Verification items for the finished model (mm, model axes). A direction names the side the tool comes from. Round coordinates to 2 decimals unless told otherwise and drop trailing zeros. Order: outer loops, then holes, each group sorted by start corner. A loop starts at its lowest first (then second) coordinate and runs counter-clockwise, first axis right, second up. Notation, with made-up numbers: (47, 0) -> (79, 0) arc R32 cw to (79, 28) -> close; hole circle Ø2 at (-12.75, 42). An arc over 180 degrees is marked (long way). Put each result on its own line as item: value.
```python
from build123d import *

# Parameters (mm, degrees)
CUT_EXTRUDE_1_DEPTH = 80.296910406
CUT_EXTRUDE_2_DEPTH = 4


with BuildPart() as part:
    # Sketch 1 → Revolve 1 (revolve)
    with BuildSketch(Plane.XY, mode=Mode.PRIVATE) as revolve_1_sk:
        with BuildLine():
            Line((9, 8), (2.5, 8))
            Line((2.5, 8), (2.5, 0))
            Line((2.5, 0), (56, 0))
            Line((56, 0), (56, 0.4))
            ThreePointArc((56, 0.4), (54.4, 2), (56, 3.6))
            Line((56, 3.6), (56, 4))
            Line((56, 4), (9, 4))
            Line((9, 4), (9, 8))
        make_face()
    revolve(revolve_1_sk.sketch.rotate(Axis((0, 4, 0), (0, 1, 0)), 90), axis=Axis((0, 4, 0), (0, 1, 0)))

    # Sketch 2 → Cut-Extrude 1 (cut, through all)
    with BuildSketch(Plane(origin=(0, 4, 0), x_dir=(1, 0, 0), z_dir=(0, 1, 0))):
        with BuildLine():
            ThreePointArc((24.385885739, -45.927427282), (40.999913751, -31.984481744), (50.480932382, -12.476997468))
            Line((50.480932382, -12.476997468), (8.559508647, 2.781152949))
            Line((8.559508647, 2.781152949), (24.385885739, -45.927427282))
        make_face()
        with BuildLine():
            ThreePointArc((-36.143925877, -37.384711076), (-17.749379666, -48.876983555), (3.733136252, -51.865823947))
            Line((3.733136252, -51.865823947), (5.290067271, -7.281152949))
            Line((5.290067271, -7.281152949), (-36.143925877, -37.384711076))
        make_face()
        with BuildLine():
            Line((-5.290067271, -7.281152949), (-46.724060418, 22.822405177))
            ThreePointArc((-46.724060418, 22.822405177), (-51.969633664, 1.776844639), (-48.173727294, -19.577844585))
            Line((-48.173727294, -19.577844585), (-5.290067271, -7.281152949))
        make_face()
        with BuildLine():
            Line((-8.559508647, 2.781152949), (7.266868446, 51.48973318))
            ThreePointArc((7.266868446, 51.48973318), (-14.369620321, 49.975133935), (-33.506137084, 39.766050567))
            Line((-33.506137084, 39.766050567), (-8.559508647, 2.781152949))
        make_face()
        with BuildLine():
            Line((27.465795744, 44.154615434), (0, 9))
            Line((0, 9), (51.215232109, 9))
            ThreePointArc((51.215232109, 9), (43.0887199, 29.109486725), (27.465795744, 44.154615434))
        make_face()
    extrude(amount=-CUT_EXTRUDE_1_DEPTH, mode=Mode.SUBTRACT)

    # Sketch 3 → Cut-Extrude 2 (cut)
    with BuildSketch(Plane(origin=(0, 8, 0), x_dir=(1, 0, 0), z_dir=(0, 1, 0))):
        Polygon((0, 7), (-6.062177826, 3.5), (-6.062177826, -3.5), (0, -7), (6.062177826, -3.5), (6.062177826, 3.5), align=None)
    extrude(amount=-CUT_EXTRUDE_2_DEPTH, mode=Mode.SUBTRACT)


solid = part.part
```
Item 1: Depth check by flat-ended pin: pin 1 Ø2 at (y, z) = (3, 8) entering from -X; pin 2 Ø3 at (y, z) = (5, 0.5) entering from -X; pin 3 Ø2 at (y, z) = (5.5, -1.5) entering from +X. Enter the tip coordinate at first touch or a pass-through.
Geometry check:
pin 1: x = -55.54
pin 2: x = -56
pin 3: x = 8.99
Item 2: Tool access check on faces 4 (the face through (-1, 0, -13)), 5 (the face through (-6.062, 6, 0)), 6 (the face through (25, 2, -9)). Record the directions out of +Z, -Z, +X, -X, +Y, -Y that give a thin tool (end or side, any length) a straight path to the whole face; none if there is none.
Geometry check:
face 4: +Z, -Z, +X, -X, -Y
face 5: +Y
face 6: +Y, -Y
Item 3: Material ranges on line 1 along X through (y, z) = (2.75, 26); line 2 along Z through (x, y) = (38, 1.5); line 3 along Y through (x, z) = (46, -26), recorded low to high.
Geometry check:
line 1: -48 to -20.47, 4.64 to 17.91, 45.03 to 48
line 2: -39.04 to -35.5, -9 to 7.93, 35.5 to 39.04
line 3: 0 to 4
Item 4: Sectioned sample at B-B, the plane z = 0. Record the boundary of the cut face in (x, y).
Geometry check:
outline: (-56, 0) -> (-52, 0) -> (-52, 4) -> (-56, 4) -> (-56, 3.6) arc R1.6 cw to (-56, 0.4) -> close; (-15.31, 0) -> (-2.5, 0) -> (-2.5, 4) -> (-6.06, 4) -> (-6.06, 8) -> (-9, 8) -> (-9, 4) -> (-15.31, 4) -> close; (2.5, 0) -> (9.46, 0) -> (9.46, 4) -> (9, 4) -> (9, 8) -> (6.06, 8) -> (6.06, 4) -> (2.5, 4) -> close; (16.2, 0) -> (56, 0) -> (56, 0.4) arc R1.6 cw to (56, 3.6) -> (56, 4) -> (16.2, 4) -> close
Item 5: Sectioned sample at C-C, the plane x = 11. Give the number of separate pieces and of enclosed holes in the cut face, then the cut area to 3 significant figures.
Geometry check:
separate pieces: 3
enclosed holes: 0
area: 348 mm2
Item 6: Release check for a two-part mould opening along Z. For faces 1 (the face through (8, 4, -8)), 2 (the face through (49.68, 3.8, -25.84)), 3 (the face through (-25.72, 2.03, -7.56)) record: pulls with the +Z half, pulls with the -Z half, needs draft (parallel to the pull), parting line crosses it, or undercut.
Geometry check:
face 1: needs draft
face 2: parting line crosses it
face 3: undercut
Item 7: Sectioned sample at A-A, the plane y = 5.25. Record the boundary of the cut face in (x, z), then the cut area to 3 significant figures.
Geometry check:
outline: circle Ø18 at (0, 0); hole (-6.06, -3.5) -> (0, -7) -> (6.06, -3.5) -> (6.06, 3.5) -> (0, 7) -> (-6.06, 3.5) -> close
area: 127 mm2
